Job drawing, mm, ordinate dimensions from the low corner. One solid piece. Give positions to 0.01 mm unless a question says otherwise; leave off trailing zeros. Write each loop counter-clockwise with the first axis right and the second up, starting at its lowest first coordinate (ties: lowest second). Pieces come first, ordered by that corner, then holes. Notation, with made-up numbers: M 64,9 L 101,9 A33 ccw 101,44 Z; hole C 23,6.5 d4. An arc over 180 degrees is marked long. Answer as CSV lines item,"result". Start each with the question number.
1) Slice it at C-C, the plane z = 6. Give the cut face in (x, y).
2) Slice it at A-A, the plane z = 65. Give the cut face in (x, y), plus the area to 3 significant figures.
3) Slice it at D-D, the plane x = 17. Give the cut face in (y, z), plus the area to 3 significant figures.
4) Mould opens along X. For the marked faces 1, 2 and 3 say: pulls with the +X half, pulls with the -X half, needs draft (parallel to the pull), parting line crosses it, or undercut.
5) Slice it at B-B, the plane y = 6.75. Give the cut face in (x, z).
6) Wall check: line 1 along X through (y, z) = (1.5, 14.5); line 2 along Z through (x, y) = (20, 1.25); line 3 along X through (y, z) = (7.5, 51). Give the ranges that are in metal, low to high. Write a range as from..to.
7) Pin check, flat tips, straight feed: pin 1 Ø1.5 at (x, y) = (26, 1.5) entering from +Z; pin 2 Ø1 at (x, y) = (10.5, 6) entering from +Z. Stop position of each tip, or through.
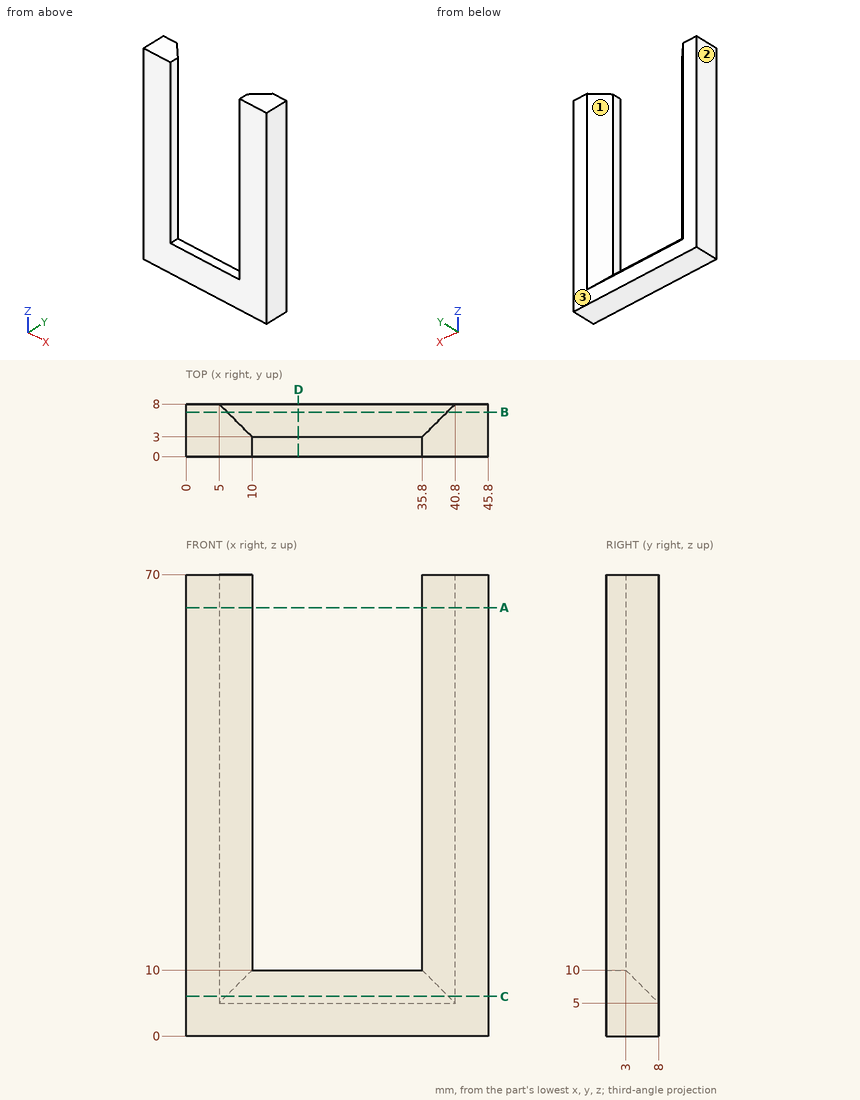
Found:
1,outline,"M 0,0 L 45.8,0 L 45.8,8 L 40.8,8 L 39.8,7 L 6,7 L 5,8 L 0,8 Z"
2,outline,"M 0,0 L 10,0 L 10,3 L 5,8 L 0,8 Z; M 35.8,0 L 45.8,0 L 45.8,8 L 40.8,8 L 35.8,3 Z"
2,area,"135 mm²"
3,outline,"M 0,0 L 8,0 L 8,5 L 3,10 L 0,10 Z"
3,area,"67.5 mm²"
4,face 1,"undercut"
4,face 2,"pulls with the -X half"
4,face 3,"needs draft"
5,outline,"M 0,0 L 45.8,0 L 45.8,70 L 39.55,70 L 39.55,6.25 L 6.25,6.25 L 6.25,70 L 0,70 Z"
6,line 1,"0..10, 35.8..45.8"
6,line 2,"0..10"
6,line 3,"0..5.5, 40.3..45.8"
7,pin 1,"z = 10"
7,pin 2,"z = 7.5"
